Could you check a few things on this drawing? It's one solid part, dimensions in mm from its lowest x, y, z. Coordinates: 2 decimals unless noted, no trailing zeros.
Item 1: I want a section at A-A (z = 1.5). Count the separate pieces of the cut face and the enclosed holes in it, and give its area (3 significant figures).
Item 2: Please list where these lines run through material, in increasing order: line 1 (X direction, y = 11.5, z = 0.95); line 2 (Y direction, x = 99.5, z = 1).
Item 3: I'm going to push a flat-ended pin straight in: P1, Ø4, axis at x = 137.668, y = 38.608, coming from the -Z side. Where does the tip first touch, or does it pass through?
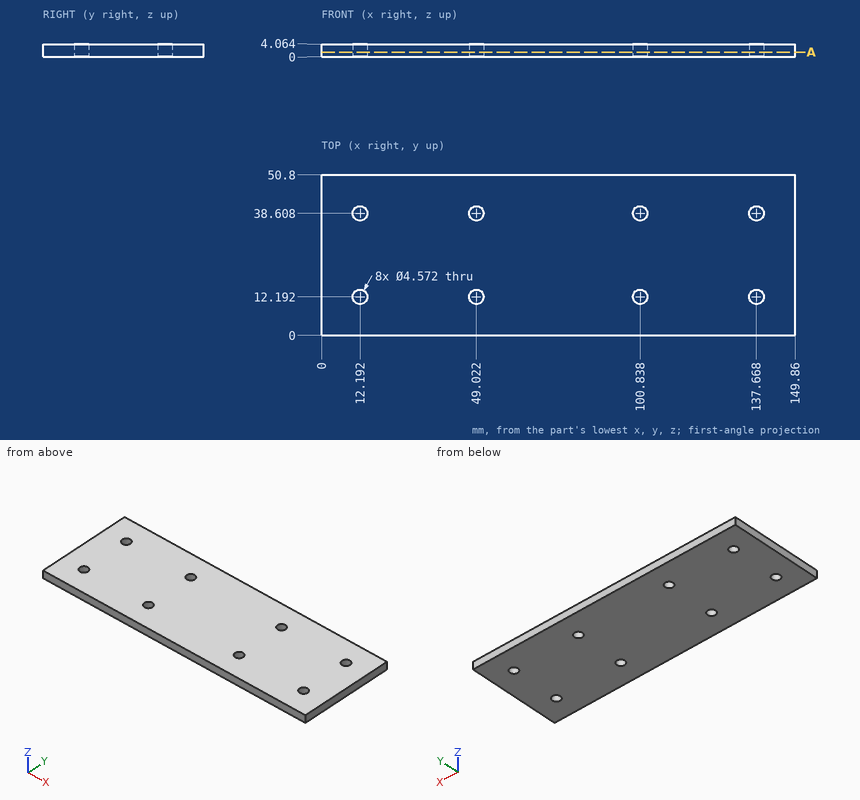
Answer:
1. separate pieces: 1
1. enclosed holes: 8
1. area: 7,480 mm2
2. line 1: x = 0 to 10.01, 14.37 to 46.84, 51.2 to 98.66, 103.02 to 135.49, 139.85 to 149.86
2. line 2: y = 0 to 10.34, 14.05 to 36.75, 40.46 to 50.8
3. P1: passes through
